Part model, mm, in its own coordinate system. Face numbers are marked on the shaded views. Give positions to 0.01 mm unless a question says otherwise; leave off trailing zeros. Order: outer loops, then holes, each group sorted by start corner. A loop starts at its lowest first (then second) coordinate and runs counter-clockwise, first axis right, second up. Notation, with made-up numbers: (34, 8) -> (60, 8) arc R20 ccw to (60, 47) -> close; hole circle Ø9 at (83.5, -6.75). An arc over 180 degrees is marked (long way). Write item = value, one per line. Start each with the question number.
Item 1: Band-saw the part on B-B on z = -230. Write the cut outline in (x, y).
Item 2: Flat gauge pins, fed straight in: P1, Ø3, axis at x = 6, z = -35, coming from the -Y side; P2, Ø12, axis at x = 221, z = -290.5, coming from the +Y side. Where does each tip first touch, or does it go through?
Item 3: Drill centre lines: line 1 along X through (y, z) = (-53.5, -259.5); line 2 along Z through (x, y) = (43.5, 89.5); line 3 along Y through (x, z) = (203.5, -296). Where is each one in solid material? Low to high.
Item 4: Band-saw the part on C-C on x = 168.5. Write the cut outline in (y, z).
Item 5: Pull direction X, two halves, no side cores. Call the marked faces 1, 2, 3 and 4: +X half, -X half, draft (parallel to the pull), parting line (faces both ways), or undercut.
Item 6: Band-saw the part on A-A on y = -2.5. Write the cut outline in (x, z), plus the area to 3 significant figures.
Item 7: Band-saw the part on D-D on z = -293. Write the cut outline in (x, y), plus the area to 3 significant figures.
```python
from build123d import *

# Parameters (mm, degrees)
BOSS_EXTRUDE1_DEPTH  = 350
SKETCH4_W            = 400
SKETCH4_H            = 330
CUT_EXTRUDE1_DEPTH   = 21.5
SKETCH5_W            = 130
SKETCH5_H            = 130
CUT_EXTRUDE2_DEPTH   = 30
FILLET1_R            = 5
SKETCH15_W           = 130
SKETCH15_H           = 10
CUT_EXTRUDE3_DEPTH   = 25
SKETCH16_W           = 130
SKETCH16_H           = 10
BOSS_EXTRUDE6_DEPTH  = 25
SKETCH22_W           = 130
SKETCH22_H           = 130
BOSS_EXTRUDE11_DEPTH = 10
BOSS_EXTRUDE12_DEPTH = 10
CUT_EXTRUDE4_DEPTH   = 10


with BuildPart() as part:
    # Sketch3 → Boss-Extrude1 (new body)
    with BuildSketch(Plane.XY):
        Polygon((-76.099744246, 110.652173913), (343.900255754, 110.652173913), (343.900255754, -79.347826087), (323.900255754, -79.347826087), (323.900255754, 79.152173913), (-56.099744246, 79.152173913), (-56.099744246, -79.347826087), (-76.099744246, -79.347826087), align=None)
    extrude(amount=-BOSS_EXTRUDE1_DEPTH)

    # Sketch4 → Cut-Extrude1 (cut)
    with BuildSketch(Plane(origin=(0, 110.652173913, 0), x_dir=(1, 0, 0), z_dir=(0, 1, 0))):
        with Locations((133.900255754, 175)):
            Rectangle(SKETCH4_W, SKETCH4_H)
    extrude(amount=-CUT_EXTRUDE1_DEPTH, mode=Mode.SUBTRACT)

    # Sketch5 → Cut-Extrude2 (cut)
    with BuildSketch(Plane(origin=(0, 89.152173913, 0), x_dir=(1, 0, 0), z_dir=(0, 1, 0))):
        with Locations((33.900255754, 110)):
            Rectangle(SKETCH5_W, SKETCH5_H)
        with BuildLine():
            Line((-21.099744246, 247.552781264), (88.900255754, 247.552781264))
            ThreePointArc((88.900255754, 247.552781264), (98.900255754, 237.552781264), (88.900255754, 227.552781264))
            Line((88.900255754, 227.552781264), (-21.099744246, 227.552781264))
            ThreePointArc((-21.099744246, 227.552781264), (-31.099744246, 237.552781264), (-21.099744246, 247.552781264))
        make_face()
        with BuildLine():
            Line((-21.099744246, 315.266550997), (88.900255754, 315.266550997))
            ThreePointArc((88.900255754, 315.266550997), (98.900255754, 305.266550997), (88.900255754, 295.266550997))
            Line((88.900255754, 295.266550997), (-21.099744246, 295.266550997))
            ThreePointArc((-21.099744246, 295.266550997), (-31.099744246, 305.266550997), (-21.099744246, 315.266550997))
        make_face()
    extrude(amount=-CUT_EXTRUDE2_DEPTH, mode=Mode.SUBTRACT)

    # Fillet1
    fillet1_edges = [part.edges().sort_by_distance(p)[0] for p in [
        (-76.099744246, 110.652173913, -175),
        (343.900255754, 110.652173913, -175),
    ]]
    fillet(fillet1_edges, radius=FILLET1_R)

    # Sketch15 → Cut-Extrude3 (cut)
    with BuildSketch(Plane.XY.offset(-175)):
        with Locations((33.900255754, 84.152173913)):
            Rectangle(SKETCH15_W, SKETCH15_H)
    extrude(amount=-CUT_EXTRUDE3_DEPTH, mode=Mode.SUBTRACT)

    # Sketch16 → Boss-Extrude6 (add)
    with BuildSketch(Plane(origin=(0, 0, -45), x_dir=(-1, 0, 0), z_dir=(0, 0, -1))):
        with Locations((-33.900255754, 84.152173913)):
            Rectangle(SKETCH16_W, SKETCH16_H)
    extrude(amount=BOSS_EXTRUDE6_DEPTH)

    # Sketch22 → Boss-Extrude11 (add)
    with BuildSketch(Plane(origin=(0, 89.152173913, 0), x_dir=(1, 0, 0), z_dir=(0, 1, 0))):
        with Locations((33.900255754, 135)):
            Rectangle(SKETCH22_W, SKETCH22_H)
    extrude(amount=-BOSS_EXTRUDE11_DEPTH)

    # Sketch23 → Boss-Extrude12 (add)
    with BuildSketch(Plane(origin=(0, 89.152173913, 0), x_dir=(1, 0, 0), z_dir=(0, 1, 0))):
        with BuildLine():
            ThreePointArc((-21.099744246, 295.266550997), (-31.099744246, 305.266550997), (-21.099744246, 315.266550997))
            Line((-21.099744246, 315.266550997), (88.900255754, 315.266550997))
            ThreePointArc((88.900255754, 315.266550997), (98.900255754, 305.266550997), (88.900255754, 295.266550997))
            Line((88.900255754, 295.266550997), (-21.099744246, 295.266550997))
        make_face()
        with BuildLine():
            ThreePointArc((-21.099744246, 227.552781264), (-31.099744246, 237.552781264), (-21.099744246, 247.552781264))
            Line((-21.099744246, 247.552781264), (88.900255754, 247.552781264))
            ThreePointArc((88.900255754, 247.552781264), (98.900255754, 237.552781264), (88.900255754, 227.552781264))
            Line((88.900255754, 227.552781264), (-21.099744246, 227.552781264))
        make_face()
    extrude(amount=-BOSS_EXTRUDE12_DEPTH)

    # Sketch24 → Cut-Extrude4 (cut)
    with BuildSketch(Plane(origin=(0, 89.152173913, 0), x_dir=(1, 0, 0), z_dir=(0, 1, 0))):
        with BuildLine():
            Line((0, 240), (270.518831375, 240))
            ThreePointArc((270.518831375, 240), (280.518831375, 230), (270.518831375, 220))
            Line((270.518831375, 220), (0, 220))
            ThreePointArc((0, 220), (-10, 230), (0, 240))
        make_face()
        with BuildLine():
            Line((270.518831375, 110), (0, 110))
            ThreePointArc((0, 110), (-10, 120), (0, 130))
            Line((0, 130), (270.518831375, 130))
            ThreePointArc((270.518831375, 130), (280.518831375, 120), (270.518831375, 110))
        make_face()
    extrude(amount=-CUT_EXTRUDE4_DEPTH, mode=Mode.SUBTRACT)


solid = part.part
```
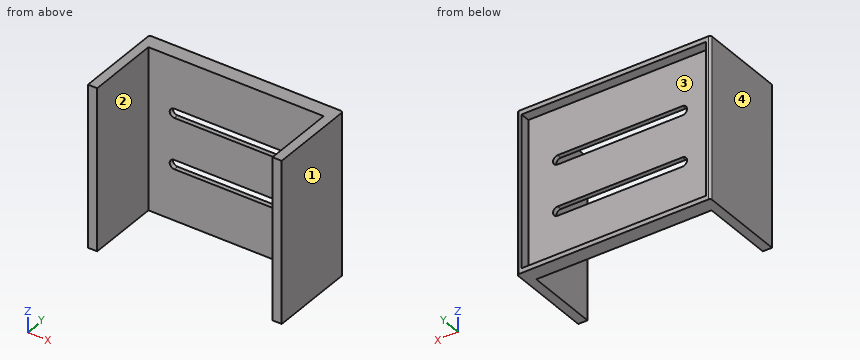
Values found:
q1.outline = (-76.1, -79.35) -> (-56.1, -79.35) -> (-56.1, 79.15) -> (-10, 79.15) -> (-10, 89.15) -> (-66.1, 89.15) -> (-66.1, 110.65) -> (-71.1, 110.65) arc R5 ccw to (-76.1, 105.65) -> close; (280.52, 79.15) -> (323.9, 79.15) -> (323.9, -79.35) -> (343.9, -79.35) -> (343.9, 105.65) arc R5 ccw to (338.9, 110.65) -> (333.9, 110.65) -> (333.9, 89.15) -> (280.52, 89.15) -> close
q2.P1 = 79.15
q2.P2 = 89.15
q3.line_1 = -76.1 to -56.1, 323.9 to 343.9
q3.line_2 = -350 to -340, -10 to 0
q3.line_3 = 79.15 to 89.15
q4.outline = (79.15, -350) -> (110.65, -350) -> (110.65, -340) -> (89.15, -340) -> (89.15, -240) -> (79.15, -240) -> close; (79.15, -220) -> (89.15, -220) -> (89.15, -130) -> (79.15, -130) -> close; (79.15, -110) -> (89.15, -110) -> (89.15, -10) -> (110.65, -10) -> (110.65, 0) -> (79.15, 0) -> close
q5.face_1 = +X half
q5.face_2 = undercut
q5.face_3 = undercut
q5.face_4 = -X half
q6.outline = (-76.1, -350) -> (-56.1, -350) -> (-56.1, 0) -> (-76.1, 0) -> close; (323.9, -350) -> (343.9, -350) -> (343.9, 0) -> (323.9, 0) -> close
q6.area = 14,000 mm^2
q7.outline = (-76.1, -79.35) -> (-56.1, -79.35) -> (-56.1, 79.15) -> (323.9, 79.15) -> (323.9, -79.35) -> (343.9, -79.35) -> (343.9, 105.65) arc R5 ccw to (338.9, 110.65) -> (333.9, 110.65) -> (333.9, 89.15) -> (-66.1, 89.15) -> (-66.1, 110.65) -> (-71.1, 110.65) arc R5 ccw to (-76.1, 105.65) -> close
q7.area = 11,000 mm^2
